Input: part model. Units: mm. Frame: model coordinates. A direction names the side the tool comes from. Coordinates: 2 decimals unless noted, no trailing zeros. Loops run counter-clockwise (first coordinate to the right, second up) from the corner with the lowest first, then second, coordinate; pieces in that order, holes last.
```python
from build123d import *

# Parameters (mm, degrees)
SKETCH1_W           = 215.9
SKETCH1_H           = 215.9
BOSS_EXTRUDE1_DEPTH = 114.3
SKETCH2_W           = 203.2
SKETCH2_H           = 203.2
CUT_EXTRUDE1_DEPTH  = 107.95
MOTOR_DRIVER_R      = 1.5875
CUT_EXTRUDE4_DEPTH  = 107.95


with BuildPart() as part:
    # Sketch1 → Boss-Extrude1 (new body)
    with BuildSketch(Plane(origin=(0, 0, 0), x_dir=(1, 0, 0), z_dir=(0, 1, 0))):
        with Locations((107.95, 107.95)):
            Rectangle(SKETCH1_W, SKETCH1_H)
    extrude(amount=BOSS_EXTRUDE1_DEPTH)

    # Sketch2 → Cut-Extrude1 (cut)
    with BuildSketch(Plane(origin=(0, 114.3, 0), x_dir=(1, 0, 0), z_dir=(0, 1, 0))):
        with Locations((107.95, 107.95)):
            Rectangle(SKETCH2_W, SKETCH2_H)
    extrude(amount=-CUT_EXTRUDE1_DEPTH, mode=Mode.SUBTRACT)

    # Motor Driver → Cut-Extrude4 (cut)
    with BuildSketch(Plane(origin=(0, 6.35, 0), x_dir=(1, 0, 0), z_dir=(0, 1, 0))):
        with Locations((37.2745, 203.5175)):
            Circle(MOTOR_DRIVER_R)
        with Locations((60.0075, 203.5175)):
            Circle(MOTOR_DRIVER_R)
        with Locations((59.8805, 91.6305)):
            Circle(MOTOR_DRIVER_R)
        with Locations((37.2745, 91.6305)):
            Circle(MOTOR_DRIVER_R)
    extrude(amount=-CUT_EXTRUDE4_DEPTH, mode=Mode.SUBTRACT)


solid = part.part
```
Item 1: Section query C-C (x = 138.5). Output: boundary loops of the cut face in (y, z), then the cut area to 3 significant figures.
Result:
outline: (0, -215.9) - (114.3, -215.9) - (114.3, -209.55) - (6.35, -209.55) - (6.35, -6.35) - (114.3, -6.35) - (114.3, 0) - (0, 0) - close
area: 2,740 mm2
Item 2: Reachability of faces 1 (the face through (107, 6.35, -109)), 2 (the face through (215.9, 56, -106)) from +Z, -Z, +X, -X, +Y, -Y: full face, straight path, thin tool, end or side. Return the list, or none.
Result:
face 1: +Y
face 2: +Z, -Z, +X, +Y, -Y
Item 3: Section query A-A (y = 90). Output: boundary loops of the cut face in (x, z), then the cut area to 3 significant figures.
Result:
outline: (0, -215.9) - (215.9, -215.9) - (215.9, 0) - (0, 0) - close; hole (6.35, -209.55) - (209.55, -209.55) - (209.55, -6.35) - (6.35, -6.35) - close
area: 5,320 mm2
Item 4: Mould query, pull axis Z, two halves, no side actions, for faces 3 (the face through (0, 56, -106)), 4 (the face through (107, 61, -6.35)), 5 (the face through (106, 56, 0)). Classes: +Z half, -Z half, draft (parallel to the pull), parting line (faces both ways), or undercut.
Result:
face 3: draft
face 4: undercut
face 5: +Z half
Item 5: Contact query for flat-ended pins moving along their axis: P1, Ø3, axis at x = 37.27, z = -203.52, coming from the -Y side; P2, Ø5, axis at x = 60.01, z = -203.52, coming from the +Y side. Output: stop coordinate, or through.
Result:
P1: passes through
P2: stops at y = 6.35
Item 6: Section query B-B (z = -156.5). Output: boundary loops of the cut face in (x, y).
Result:
outline: (0, 0) - (215.9, 0) - (215.9, 114.3) - (209.55, 114.3) - (209.55, 6.35) - (6.35, 6.35) - (6.35, 114.3) - (0, 114.3) - close
Item 7: Line query: L1, parallel to X at y = 59, z = -55.5; L2, parallel to Z at x = 55.5, y = 67.5; L3, parallel to Y at x = 107.5, z = -200.5. Output: solid intervals per line, ascending.
Result:
L1: x = 0 to 6.35, 209.55 to 215.9
L2: z = -215.9 to -209.55, -6.35 to 0
L3: y = 0 to 6.35
